from build123d import *

# Parameters (mm, degrees)
ESQUISSE1_R             = 8.5
BOSS_EXTRU_1_DEPTH      = 6
ESQUISSE2_R             = 4
BOSS_EXTRU_2_DEPTH      = 6
ENL_V_MAT_EXTRU_1_REACH = 18.985
ESQUISSE3_R             = 2.5


with BuildPart() as part:
    # Esquisse1 → Boss.-Extru.1 (new body)
    with BuildSketch(Plane(origin=(0, 0, 0), x_dir=(1, 0, 0), z_dir=(0, 1, 0))):
        with Locations(Location((0, 0, 0), (0, 0, 270))):
            Circle(ESQUISSE1_R)
    extrude(amount=BOSS_EXTRU_1_DEPTH)

    # Esquisse2 → Boss.-Extru.2 (add)
    with BuildSketch(Plane(origin=(0, 6, 0), x_dir=(1, 0, 0), z_dir=(0, 1, 0))):
        with Locations(Location((0, 0, 0), (0, 0, 270))):
            Circle(ESQUISSE2_R)
    extrude(amount=BOSS_EXTRU_2_DEPTH)

    # Esquisse3 → Enlèv. mat.-Extru.1 (cut, up to next)
    with BuildSketch(Plane(origin=(0, 12, 0), x_dir=(1, 0, 0), z_dir=(0, 1, 0)), mode=Mode.PRIVATE) as enl_v_mat_extru_1_sk1:
        with Locations(Location((0, 0, 0), (0, 0, 270))):
            Circle(ESQUISSE3_R)
    enl_v_mat_extru_1_tool1 = extrude(enl_v_mat_extru_1_sk1.sketch, amount=-ENL_V_MAT_EXTRU_1_REACH, mode=Mode.PRIVATE) & part.part
    add(enl_v_mat_extru_1_tool1.solids().sort_by_distance((0, 12, 0))[0], mode=Mode.SUBTRACT)


solid = part.part
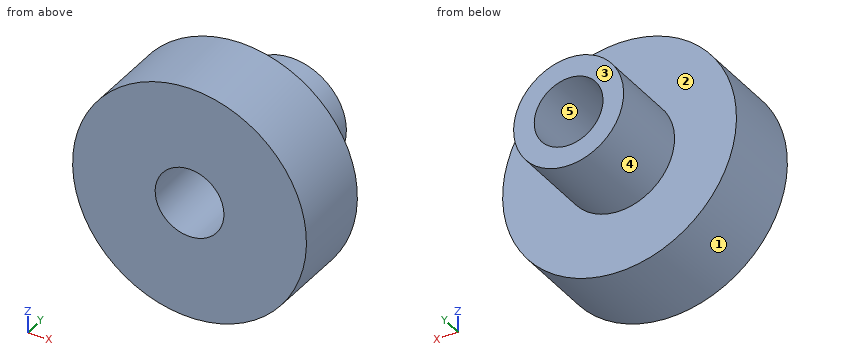
Here's how the part is built. I have some questions about the finished solid (model axes, mm). Face numbers are marked on the shaded views. A direction names the side the tool comes from. Give positions to 0.01 mm unless a question says otherwise; leave off trailing zeros. Loops run counter-clockwise (first coordinate to the right, second up) from the corner with the lowest first, then second, coordinate; pieces in that order, holes last. Notation, with made-up numbers: (64, 74.5) -> (113, 74.5) arc R15 ccw to (113, 92.5) -> close; hole circle Ø4 at (-11.75, 2.25). An arc over 180 degrees is marked (long way). Answer as a JSON object with one key per item and string values. Group by question number.
Item 1: Imagine slicing it at B-B on z = 0. Write out the boundary of the cut face in (x, y), then the cut area to 3 significant figures.
Item 2: Thinking about a two-plate mould opening in Z: for the marked faces 3, 4 and 5, which applies, pulls with the +Z half, pulls with the -Z half, needs draft (parallel to the pull), parting line crosses it, or undercut?
Item 3: On a 3-axis mill with a long thin cutter (end or side, diameter ignored), from which of +Z, -Z, +X, -X, +Y, -Y can I reach the whole of each face in a straight line? I mean the marked faces 1 and 2. Say none if no direction works.
Item 4: Imagine slicing it at C-C on y = 9.5. Write out the boundary of the cut face in (x, z), then the cut area to 3 significant figures.
Item 5: Imagine slicing it at D-D on z = -3.75. Write out the boundary of the cut face in (x, y).
Item 6: I need wall thicknesses on L1, parallel to X at y = 2.5, z = 0; L2, parallel to Y at x = -2.25, z = -4; L3, parallel to X at y = 4.25, z = 7.5. Which ranges of each line are inside material? Lowest first, please.
Item 7: Imagine slicing it at A-A on x = 0. Write out the boundary of the cut face in (y, z), then the cut area to 3 significant figures.
Item 8: Will these pins go through, and if not, where does the flat tip stop? pin 1 (1 mm diameter, centred on x = 6.5, z = -6.5, fed in from +Y); pin 2 (1 mm diameter, centred on x = 6, y = 1.5, fed in from +Z); pin 3 (2 mm diameter, centred on y = 3, z = -2.5, fed in from -X); pin 4 (3 mm diameter, centred on y = 7, z = -4.5, fed in from +X).
Answer list:
{
 "1": {"outline": "(-8.5, 0) -> (-2.5, 0) -> (-2.5, 12) -> (-4, 12) -> (-4, 6) -> (-8.5, 6) -> close; (2.5, 0) -> (8.5, 0) -> (8.5, 6) -> (4, 6) -> (4, 12) -> (2.5, 12) -> close", "area": "90.0 mm2"},
 "2": {"face 3": "needs draft", "face 4": "parting line crosses it", "face 5": "undercut"},
 "3": {"face 1": "+Y, -Y", "face 2": "+Y"},
 "4": {"outline": "circle Ø8 at (0, 0); hole circle Ø5 at (0, 0)", "area": "30.6 mm2"},
 "5": {"outline": "(-7.63, 0) -> (7.63, 0) -> (7.63, 6) -> (1.39, 6) -> (1.39, 12) -> (-1.39, 12) -> (-1.39, 6) -> (-7.63, 6) -> close"},
 "6": {"L1": "x = -8.5 to -2.5, 2.5 to 8.5", "L2": "y = 0 to 6", "L3": "x = -4 to 4"},
 "7": {"outline": "(0, -8.5) -> (6, -8.5) -> (6, -4) -> (12, -4) -> (12, -2.5) -> (0, -2.5) -> close; (0, 2.5) -> (12, 2.5) -> (12, 4) -> (6, 4) -> (6, 8.5) -> (0, 8.5) -> close", "area": "90.0 mm2"},
 "8": {"pin 1": "passes through", "pin 2": "stops at z = 6.48", "pin 3": "stops at x = -8.37", "pin 4": "stops at x = 7.8"}
}
